Check sheet for the modelled part. Datum: model origin and axes. Units: mm. A direction names the side the tool comes from. Coordinates: 2 decimals unless noted, no trailing zeros. Order: outer loops, then holes, each group sorted by start corner. A loop starts at its lowest first (then second) coordinate and runs counter-clockwise, first axis right, second up.
1. Cross-section at D-D (y = 65.5). Enter the section's corners in (x, z), then the cut area to 3 significant figures.
2. Cross-section at C-C (z = 83). Enter the section's corners in (x, y).
3. Thickness scan on line 1 (Y direction, x = -12, z = -139); line 2 (Z direction, x = -57, y = 2.5). Record the ranges inside material, lowest first.
4. Draft check along Y on faces 1 (the cylindrical face through (-6.46, 49.2, 60.61)), 2 (the flat face through (0, -12.7, -25)), 3 (the flat face through (88.9, -1, -88)). Enter one of: released by +Y, released by -Y, zero draft, split by the parting line, or undercut.
5. Set-up check for faces 4 (the flat face through (0, 12.7, -25)), 5 (the flat face through (-1, 21, -177.8)), 6 (the flat face through (38, 41, 0)): record each of +Z, -Z, +X, -X, +Y, -Y from which the full face is reachable in a straight line by a thin tool's end or side.
6. Gauge pin test, flat ends, axial feed: pin 1 Ø1 at (y, z) = (38.5, 92.5) entering from -X; pin 2 Ø1.5 at (y, z) = (-36, 2.5) entering from -X. Record the tip position at first contact, or that the pin passes through.
7. Cross-section at A-A (x = 0). Enter the section's corners in (y, z).
```python
from build123d import *

# Parameters (mm, degrees)
F0_R     = 49.624192
F1_DEPTH = 122.936
F2_W     = 177.8
F2_H     = 177.8
F3_DEPTH = 177.8
F4_W     = 25.4
F4_H     = 25.4
F5_DEPTH = 376.936


with BuildPart() as f1:
    # F0 (on Top) → F1 (new body)
    with BuildSketch(Plane.XY):
        Circle(F0_R)
    extrude(amount=F1_DEPTH)

    # F2 (on Top) → F3 (join)
    with BuildSketch(Plane.XY):
        Rectangle(F2_W, F2_H)
    extrude(amount=-F3_DEPTH)

    # F4 (on face) → F5 (cut)
    with BuildSketch(Plane.XY.offset(122.936)):
        Rectangle(F4_W, F4_H)
    extrude(amount=-F5_DEPTH, mode=Mode.SUBTRACT)


solid = f1.part
```
Data:
1. outline: (-88.9, -177.8) - (88.9, -177.8) - (88.9, 0) - (-88.9, 0) - close
1. area: 31,600 mm2
2. outline: circle Ø99.25 at (0, 0); hole (-12.7, -12.7) - (12.7, -12.7) - (12.7, 12.7) - (-12.7, 12.7) - close
3. line 1: y = -88.9 to -12.7, 12.7 to 88.9
3. line 2: z = -177.8 to 0
4. face 1: split by the parting line
4. face 2: undercut
4. face 3: zero draft
5. face 4: +Z, -Z
5. face 5: -Z, +X, -X, +Y, -Y
5. face 6: +Z
6. pin 1: stops at x = -31.91
6. pin 2: stops at x = -34.93
7. outline: (-88.9, -177.8) - (-12.7, -177.8) - (-12.7, 122.94) - (-49.62, 122.94) - (-49.62, 0) - (-88.9, 0) - close; (12.7, -177.8) - (88.9, -177.8) - (88.9, 0) - (49.62, 0) - (49.62, 122.94) - (12.7, 122.94) - close
